Build history of the part. All positions in model axes, mm. A direction names the side the tool comes from. Give positions to 0.01 mm unless a question says otherwise; leave off trailing zeros. Order: outer loops, then holes, each group sorted by start corner. A loop starts at its lowest first (then second) coordinate and runs counter-clockwise, first axis right, second up. Notation, with made-up numbers: M -27,-17.75 L -5,-17.75 A19 cw -5,17.25 Z; hole C 77.5,48 d8. An arc over 180 degrees is marked long. Use CSV: the item, a comma, the result in double quotes. Start each with the question number.
Item 1: Band-saw the part on C-C on z = -208. Write the cut outline in (x, y), plus the area to 3 significant figures.
Item 2: Which spindle directions (+Z, -Z, +X, -X, +Y, -Y) get a long thin tool onto all of the face, cutting with end or side? Do faces 4 (the flat face through (197, 15, -55)), 5 (the flat face through (197, 17, -55)). Say none if no direction does.
Item 3: Band-saw the part on B-B on x = 280. Write the cut outline in (y, z), plus the area to 3 significant figures.
Item 4: Two-plate mould, pull along X, no slides. Class faces 1 (the flat face through (402, 8, -49)), 2 (the flat face through (400, 7, -49)), 3 (the flat face through (-2, 8, -49)): pulls with the +X half, pulls with the -X half, needs draft (parallel to the pull), parting line crosses it, or undercut.
Item 5: Band-saw the part on A-A on y = 6.25. Write the cut outline in (x, z).
Item 6: Wall check: line 1 along X through (y, z) = (5.5, -92); line 2 along Z through (x, y) = (59, 14); line 3 along Y through (x, z) = (373.5, 76). Give the ranges that are in metal, low to high.
from build123d import *

# Parameters (mm, degrees)
SKETCH1_W           = 404
SKETCH1_H           = 404
SKETCH1_W_2         = 400
SKETCH1_H_2         = 400
BOSS_EXTRUDE1_DEPTH = 15
SKETCH3_W           = 404
SKETCH3_H           = 404
BOSS_EXTRUDE2_DEPTH = 2


with BuildPart() as part:
    # Sketch1 → Boss-Extrude1 (new body)
    with BuildSketch(Plane(origin=(0, 0, 0), x_dir=(1, 0, 0), z_dir=(0, 1, 0))):
        with Locations((200, 52.080415622)):
            Rectangle(SKETCH1_W, SKETCH1_H)
        with Locations((200, 52.080415622)):
            Rectangle(SKETCH1_W_2, SKETCH1_H_2, mode=Mode.SUBTRACT)
    extrude(amount=BOSS_EXTRUDE1_DEPTH)

    # Sketch3 → Boss-Extrude2 (add)
    with BuildSketch(Plane(origin=(0, 15, 0), x_dir=(1, 0, 0), z_dir=(0, 1, 0))):
        with Locations((200, 52.080415622)):
            Rectangle(SKETCH3_W, SKETCH3_H)
    extrude(amount=BOSS_EXTRUDE2_DEPTH)


solid = part.part
Model answer:
1,outline,"M -2,0 L 0,0 L 0,15 L 400,15 L 400,0 L 402,0 L 402,17 L -2,17 Z"
1,area,"868 mm^2"
2,face 4,"-Y"
2,face 5,"+Z, -Z, +X, -X, +Y"
3,outline,"M 0,-254.08 L 17,-254.08 L 17,149.92 L 0,149.92 L 0,147.92 L 15,147.92 L 15,-252.08 L 0,-252.08 Z"
3,area,"868 mm^2"
4,face 1,"pulls with the +X half"
4,face 2,"undercut"
4,face 3,"pulls with the -X half"
5,outline,"M -2,-254.08 L 402,-254.08 L 402,149.92 L -2,149.92 Z; hole M 0,-252.08 L 400,-252.08 L 400,147.92 L 0,147.92 Z"
6,line 1,"x = -2 to 0, 400 to 402"
6,line 2,"z = -254.08 to -252.08, 147.92 to 149.92"
6,line 3,"y = 15 to 17"
